The drawing under review shows one solid part. Ordinate dimensions are in mm from its lowest x, y, z. Coordinates: 2 decimals unless noted, no trailing zeros. Write each loop counter-clockwise with the first axis right and the second up, starting at its lowest first coordinate (ties: lowest second). Pieces come first, ordered by that corner, then holes.
1) We need section B-B on y = 25. Write out the cut boundary in (x, z).
2) We need section C-C on z = 0.45. Write out the cut boundary in (x, y).
3) To check wall thickness, follow line 1 along Y through (x, z) = (35, 0.75); line 2 along X through (y, z) = (54.5, 0.9); line 3 along Y through (x, z) = (7, 0.8). State the ranges of each line that lie inside material, in increasing order.
4) We need section A-A on x = 35. Write out the cut boundary in (y, z), then the cut area to 3 significant figures.
5) Insertion check: P1, Ø6.5, axis at x = 35, y = 25, coming from the +Z side; P2, Ø4.5, axis at x = 35, y = 55, coming from the -Z side. Each pin has a flat end and moves straight along its axis. Give the tip position at first contact, or say it passes through.
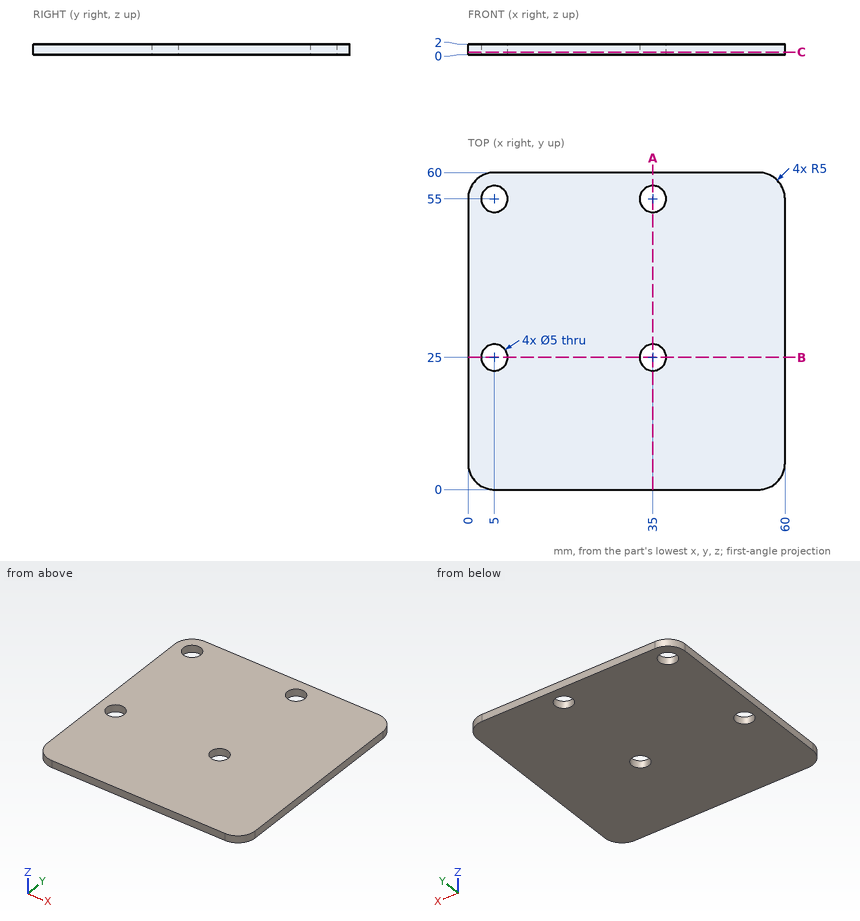
Result:
1. outline: (0, 0) - (2.5, 0) - (2.5, 2) - (0, 2) - close; (7.5, 0) - (32.5, 0) - (32.5, 2) - (7.5, 2) - close; (37.5, 0) - (60, 0) - (60, 2) - (37.5, 2) - close
2. outline: (0, 5) arc R5 ccw to (5, 0) - (55, 0) arc R5 ccw to (60, 5) - (60, 55) arc R5 ccw to (55, 60) - (5, 60) arc R5 ccw to (0, 55) - close; hole circle Ø5 at (5, 25); hole circle Ø5 at (5, 55); hole circle Ø5 at (35, 25); hole circle Ø5 at (35, 55)
3. line 1: y = 0 to 22.5, 27.5 to 52.5, 57.5 to 60
3. line 2: x = 0 to 2.55, 7.45 to 32.55, 37.45 to 60
3. line 3: y = 0 to 23.5, 26.5 to 53.5, 56.5 to 60
4. outline: (0, 0) - (22.5, 0) - (22.5, 2) - (0, 2) - close; (27.5, 0) - (52.5, 0) - (52.5, 2) - (27.5, 2) - close; (57.5, 0) - (60, 0) - (60, 2) - (57.5, 2) - close
4. area: 100 mm2
5. P1: stops at z = 2
5. P2: passes through
